```python
from build123d import *

# Parameters (mm, degrees)
SKETCH1_R           = 6.5
SKETCH1_R_2         = 4
BOSS_EXTRUDE1_DEPTH = 20
BOSS_EXTRUDE2_START = 62
SKETCH2_R           = 6.5
BOSS_EXTRUDE2_DEPTH = 62
SKETCH3_W           = 4
SKETCH3_H           = 12.369316876
BOSS_EXTRUDE3_DEPTH = 20
FILLET1_R           = 4
SKETCH4_R           = 2.5
CUT_EXTRUDE1_DEPTH  = 4


with BuildPart() as part:
    # Sketch1 → Boss-Extrude1 (new body)
    with BuildSketch(Plane.XY):
        Circle(SKETCH1_R)
        Circle(SKETCH1_R_2, mode=Mode.SUBTRACT)
    extrude(amount=BOSS_EXTRUDE1_DEPTH)

    # Sketch2 → Boss-Extrude2 (add)
    with BuildSketch(Plane(origin=(0, 0, 0), x_dir=(-1, 0, 0), z_dir=(0, 0, -1)).offset(BOSS_EXTRUDE2_START)):
        Circle(SKETCH2_R)
    extrude(amount=-BOSS_EXTRUDE2_DEPTH)

    # Sketch3 → Boss-Extrude3 (add)
    with BuildSketch(Plane(origin=(0, 0, -62), x_dir=(-1, 0, 0), z_dir=(0, 0, -1))):
        Rectangle(SKETCH3_W, SKETCH3_H)
    extrude(amount=BOSS_EXTRUDE3_DEPTH)

    # Fillet1
    fillet1_edges = [part.edges().sort_by_distance(p)[0] for p in [
        (0, 6.184658438, -82),
        (0, -6.184658438, -82),
    ]]
    fillet(fillet1_edges, radius=FILLET1_R)

    # Sketch4 → Cut-Extrude1 (cut)
    with BuildSketch(Plane(origin=(2, 0, 0), x_dir=(0, 0, -1), z_dir=(1, 0, 0))):
        with Locations((77, 0)):
            Circle(SKETCH4_R)
    extrude(amount=-CUT_EXTRUDE1_DEPTH, mode=Mode.SUBTRACT)


solid = part.part
```
CAD build for the part. Positions are in the model's coordinates, mm. A direction names the side the tool comes from. Coordinates: 2 decimals unless noted, no trailing zeros. Write each loop counter-clockwise with the first axis right and the second up, starting at its lowest first coordinate (ties: lowest second). Pieces come first, ordered by that corner, then holes.
(1) Flat gauge pins, fed straight in: pin 1 (4 mm diameter, centred on y = 0, z = -77, fed in from -X); pin 2 (5 mm diameter, centred on x = -3.5, z = -22, fed in from -Y); pin 3 (1.2 mm diameter, centred on x = 0.5, z = -68.5, fed in from +Y); pin 4 (1.2 mm diameter, centred on x = 0.5, z = -73.5, fed in from -Y). Where does each tip first touch, or does it go through?
(2) Cut at B-B, the plane y = 0. List the corners of the cut face in (x, z), and give its area (3 significant figures).
(3) Cut at A-A, the plane z = -77. List the corners of the cut face in (x, y).
(4) Cut at C-C, the plane x = 0. List the corners of the cut face in (y, z), and give its area (3 significant figures).
(5) Two-plate mould, pull along Y, no slides. Class faces 5 (the face through (-0.867, -3.905, 9.86)), 6 (the face through (-0.03, 5.04, -80.8)), 7 (the face through (-0.03, -5.04, -80.8)): +Y half, -Y half, draft (parallel to the pull), parting line (faces both ways), or undercut.
(6) 3-axis set-ups, long thin cutter, end or side, ignore diameter. For faces 1 (the face through (0, 0, 0)), 2 (the face through (-4, 0, -62)), 3 (the face through (4, 0, -62)), 4 (the face through (0, -6.185, -70)): which of +Z, -Z, +X, -X, +Y, -Y reach the whole face in a straight line?
(7) Cut at D-D, the plane z = -28. List the corners of the cut face in (x, y).
(8) Drill centre lines: probe 1 along Y at (x, z) = (-0.4, -77); probe 2 along Y at (x, z) = (0, 12.25); probe 3 along Z at (x, y) = (2.5, 2). Where is each one in solid material? Low to high.
Geometry says:
1. pin 1: passes through
1. pin 2: stops at y = -6.42
1. pin 3: stops at y = 6.18
1. pin 4: stops at y = -6.18
2. outline: (-6.5, -62) - (-2, -62) - (-2, -74.5) - (2, -74.5) - (2, -62) - (6.5, -62) - (6.5, 20) - (4, 20) - (4, 0) - (-4, 0) - (-4, 20) - (-6.5, 20) - close; (-2, -82) - (2, -82) - (2, -79.5) - (-2, -79.5) - close
2. area: 966 mm2
3. outline: (-2, -6.18) - (2, -6.18) - (2, -2.5) - (-2, -2.5) - close; (-2, 2.5) - (2, 2.5) - (2, 6.18) - (-2, 6.18) - close
4. outline: (-6.5, -62) - (-6.18, -62) - (-6.18, -78) arc R4 ccw to (-2.18, -82) - (2.18, -82) arc R4 ccw to (6.18, -78) - (6.18, -62) - (6.5, -62) - (6.5, 20) - (4, 20) - (4, 0) - (-4, 0) - (-4, 20) - (-6.5, 20) - close; hole circle Ø5 at (0, -77)
4. area: 1,130 mm2
5. face 5: undercut
5. face 6: +Y half
5. face 7: -Y half
6. face 1: +Z
6. face 2: -Z, -X, +Y, -Y
6. face 3: -Z, +X, +Y, -Y
6. face 4: -Z, +X, -X, -Y
7. outline: circle Ø13 at (0, 0)
8. probe 1: y = -6.18 to -2.5, 2.5 to 6.18
8. probe 2: y = -6.5 to -4, 4 to 6.5
8. probe 3: z = -62 to 0
